Autodesk Fusion 360 part; units mm, degrees
sketch "Sketch1" plane through (0, 0, 0) normal (0, 1, 0) x (1, 0, 0)
  line L0 (0, 0) -> (0, -20)
  line L1 (0, -20) -> (16, -20)
  line L2 (16, -20) -> (16, 0)
  line L3 (16, 0) -> (13, 0)
  line L4 (13, 0) -> (13, -17)
  line L5 (13, -17) -> (3, -17)
  line L6 (3, -17) -> (3, 0)
  line L7 (3, 0) -> (0, 0)
extrude "Extrude1" add sketch "Sketch1" along normal blind 60
sketch "Sketch2" plane through (0, 0, 0) normal (0, -1, 0) x (1, 0, 0)
  line L0 (0, 0) -> (3, 0)
  line L1 (3, 0) -> (3, 17)
  line L2 (3, 17) -> (13, 17)
  line L3 (13, 17) -> (13, 0)
  line L4 (13, 0) -> (16, 0)
  line L5 (16, 0) -> (16, 20)
  line L6 (16, 20) -> (0, 20)
  line L7 (0, 20) -> (0, 0)
  line L8 (16, 0) -> (66, 0)
  line L9 (66, 0) -> (66, 85)
  line L10 (66, 85) -> (146, 85)
  line L11 (146, 85) -> (146, 0)
  line L12 (146, 0) -> (166, 0)
  line L13 (166, 0) -> (166, 205)
  line L14 (166, 205) -> (46, 205)
  line L15 (46, 205) -> (46, 20)
  line L16 (46, 20) -> (16, 20)
  dimension "d3" = 50
  dimension "d4" = 85
  dimension "d5" = 80
  dimension "d6" = 20
  dimension "d7" = 205
  dimension "d8" = 120
  dimension "d9" = 185
extrude "Extrude2" add sketch "Sketch2" against normal blind 3 contours L5 L8 L9 L10 L11 L12 L13 L14 L15 L16
sketch "Sketch3" plane through (0, 0, 0) normal (0, 1, 0) x (1, 0, 0)
  line L0 (65, 0) -> (150, 0)
  line L1 (150, 0) -> (150, -10)
  line L2 (150, -10) -> (65, -10)
  line L3 (65, -10) -> (65, 0)
extrude "Extrude3" add sketch "Sketch3" along normal blind 3
sketch "Sketch4" plane through (0, 0, 0) normal (0, 1, 0) x (1, 0, 0)
sketch "Sketch5" plane through (0, 0, 0) normal (0, 0, 1) x (1, 0, 0)
  line L0 (16, 3) -> (16, 30)
  line L1 (16, 30) -> (43, 3)
  line L2 (43, 3) -> (16, 3)
extrude "Extrude4" add sketch "Sketch5" along normal blind 3
sketch "Sketch6" plane through (0, 0, 0) normal (0, -1, 0) x (1, 0, 0)
  line L0 (66, 10) -> (66, 85)
  line L1 (66, 85) -> (146, 85)
  line L2 (146, 85) -> (146, 10)
  line L3 (146, 10) -> (66, 10)
  line L4 (13, 0) -> (166, 0)
  line L5 (166, 0) -> (166, 205)
  line L6 (166, 205) -> (46, 205)
  line L7 (46, 205) -> (46, 20)
  line L8 (46, 20) -> (16, 20)
  line L9 (16, 20) -> (0, 20)
  line L10 (0, 20) -> (0, 0)
  line L11 (0, 0) -> (3, 0)
  line L12 (3, 0) -> (3, 17)
  line L13 (3, 17) -> (13, 17)
  line L14 (13, 17) -> (13, 0)
  circle A0 centre (51.25, 199.75) radius 2.25
  circle A1 centre (160.75, 199.75) radius 2.25
  circle A2 centre (51.25, 90.25) radius 2.25
  circle A3 centre (160.75, 90.25) radius 2.25
  dimension "d16" = 4.5
  dimension "d17" = 5.25
  dimension "d18" = 5.25
  dimension "d19" = 4.5
  dimension "d20" = 5.25
  dimension "d21" = 5.25
  dimension "d22" = 4.5
  dimension "d23" = 5.25
  dimension "d24" = 114.75
  dimension "d25" = 4.5
  dimension "d26" = 5.25
  dimension "d27" = 114.75
extrude "Extrude5" cut sketch "Sketch6" against normal blind 5 contours A0 | A1 | A2 | A3
sketch "Sketch7" plane through (0, 0, 0) normal (0, -1, 0) x (1, 0, 0)
  circle A0 centre (160.75, 90.25) radius 2.25
  circle A1 centre (160.75, 199.75) radius 2.25
  circle A2 centre (51.25, 90.25) radius 2.25
  circle A3 centre (51.25, 199.75) radius 2.25
  line L0 (66, 10) -> (66, 85)
  line L1 (66, 85) -> (146, 85)
  line L2 (146, 85) -> (146, 10)
  line L3 (146, 10) -> (66, 10)
  line L4 (13, 0) -> (166, 0)
  line L5 (166, 0) -> (166, 205)
  line L6 (166, 205) -> (46, 205)
  line L7 (46, 205) -> (46, 20)
  line L8 (46, 20) -> (16, 20)
  line L9 (16, 20) -> (0, 20)
  line L10 (0, 20) -> (0, 0)
  line L11 (0, 0) -> (3, 0)
  line L12 (3, 0) -> (3, 17)
  line L13 (3, 17) -> (13, 17)
  line L14 (13, 17) -> (13, 0)
  line L15 (51, 185) -> (67, 201)
  line L16 (67, 201) -> (145, 201)
  line L17 (145, 201) -> (160.9711, 185.0289)
  line L18 (160.9711, 185.0289) -> (160.9711, 107.0289)
  line L19 (51, 185) -> (51, 107)
  line L20 (51, 107) -> (66.9997, 91.0003)
  line L21 (66.9997, 91.0003) -> (144.9997, 91.0003)
  line L22 (144.9997, 91.0003) -> (160.9711, 107.0289)
  dimension "d30" = 78
  dimension "d31" = 22.627
  dimension "d32" = 78
  dimension "d33" = 78
extrude "Extrude6" cut sketch "Sketch7" against normal blind 10 contours L15 L16 L17 L18 L19 L20 L21 L22
sketch "Sketch8" plane through (0, 0, 0) normal (0, -1, 0) x (1, 0, 0)
  line L0 (66.9997, 91.0003) -> (51, 107)
  line L1 (51, 107) -> (51, 185)
  line L2 (51, 185) -> (67, 201)
  line L3 (67, 201) -> (145, 201)
  line L4 (145, 201) -> (160.9711, 185.0289)
  line L5 (160.9711, 185.0289) -> (160.9711, 107.0289)
  line L6 (160.9711, 107.0289) -> (144.9997, 91.0003)
  line L7 (144.9997, 91.0003) -> (66.9997, 91.0003)
  circle A0 centre (160.75, 90.25) radius 2.25
  circle A1 centre (160.75, 199.75) radius 2.25
  circle A2 centre (51.25, 90.25) radius 2.25
  line L8 (66, 10) -> (66, 85)
  line L9 (66, 85) -> (146, 85)
  line L10 (146, 85) -> (146, 10)
  line L11 (146, 10) -> (66, 10)
  line L12 (13, 0) -> (166, 0)
  line L13 (166, 0) -> (166, 205)
  line L14 (166, 205) -> (46, 205)
  line L15 (46, 205) -> (46, 20)
  line L16 (46, 20) -> (16, 20)
  line L17 (16, 20) -> (0, 20)
  line L18 (0, 20) -> (0, 0)
  line L19 (0, 0) -> (3, 0)
  line L20 (3, 0) -> (3, 17)
  line L21 (3, 17) -> (13, 17)
  line L22 (13, 17) -> (13, 0)
sketch "Sketch9" plane through (0, 0, 0) normal (0, -1, 0) x (1, 0, 0)
  circle A0 centre (51, 200) radius 3.6056
extrude "Extrude7" add sketch "Sketch9" against normal blind 3
sketch "Sketch10" plane through (0, 0, 0) normal (0, -1, 0) x (1, 0, 0)
  circle A0 centre (53.5, 197.5) radius 2.25
  line L0 (46, 205) -> (46, 20)
  line L1 (166, 205) -> (46, 205)
  dimension "d38" = 4.5
  dimension "d39" = 7.5
  dimension "d40" = 7.5
sketch "Sketch11" plane through (0, 0, 0) normal (0, -1, 0) x (1, 0, 0)
  circle A0 centre (160, 200) radius 4.464
extrude "Extrude8" add sketch "Sketch11" against normal blind 3
sketch "Sketch12" plane through (0, 0, 0) normal (0, -1, 0) x (1, 0, 0)
  circle A0 centre (158.5, 197.5) radius 2.25
  line L0 (166, 0) -> (166, 205)
  line L1 (166, 205) -> (46, 205)
  dimension "d43" = 4.5
  dimension "d44" = 7.5
  dimension "d45" = 7.5
extrude "Extrude9" cut sketch "Sketch10" against normal blind 3
extrude "Extrude10" cut sketch "Sketch12" against normal blind 3
sketch "Sketch13" plane through (0, 0, 0) normal (0, -1, 0) x (1, 0, 0)
  circle A0 centre (50, 90) radius 3.5652
  circle A1 centre (160, 90) radius 4.4009
extrude "Extrude11" add sketch "Sketch13" against normal blind 3 contours A0
extrude "Extrude12" add sketch "Sketch8" against normal blind 3 contours A0
sketch "Sketch14" plane through (0, 0, 0) normal (0, -1, 0) x (1, 0, 0)
  circle A0 centre (158.5, 197.5) radius 2.25
  circle A1 centre (53.5, 197.5) radius 2.25
  line L0 (66.9997, 91.0003) -> (51, 107)
  line L1 (51, 107) -> (51, 185)
  line L2 (51, 185) -> (67, 201)
  line L3 (67, 201) -> (145, 201)
  line L4 (145, 201) -> (160.9711, 185.0289)
  line L5 (160.9711, 185.0289) -> (160.9711, 107.0289)
  line L6 (160.9711, 107.0289) -> (144.9997, 91.0003)
  line L7 (144.9997, 91.0003) -> (66.9997, 91.0003)
  line L8 (66, 10) -> (66, 85)
  line L9 (66, 85) -> (146, 85)
  line L10 (146, 85) -> (146, 10)
  line L11 (146, 10) -> (66, 10)
  line L12 (13, 0) -> (166, 0)
  line L13 (166, 0) -> (166, 205)
  line L14 (166, 205) -> (46, 205)
  line L15 (46, 205) -> (46, 20)
  line L16 (46, 20) -> (16, 20)
  line L17 (16, 20) -> (0, 20)
  line L18 (0, 20) -> (0, 0)
  line L19 (0, 0) -> (3, 0)
  line L20 (3, 0) -> (3, 17)
  line L21 (3, 17) -> (13, 17)
  line L22 (13, 17) -> (13, 0)
  circle A2 centre (53.5, 92.5) radius 2.25
  circle A3 centre (158.5, 92.5) radius 2.25
  dimension "d54" = 4.5
  dimension "d55" = 7.5
  dimension "d57" = 7.5
  dimension "d58" = 4.5
  dimension "d59" = 7.5
  dimension "d60" = 7.5
extrude "Extrude13" cut sketch "Sketch14" against normal blind 3 contours A2 | A3
fillet "Fillet1" radius 5 1 edges at (46, 1.5, 205)
fillet "Fillet2" radius 5 1 edges at (166, 1.5, 205)
fillet "Fillet3" radius 5 1 edges at (166, 1.5, 0)
extrude "Extrude14" add 1 faces at (59.3333, 3, 38.3333) along direction (0, 1, 0) blind 2
sketch "Sketch15" plane through (0, 5, 0) normal (0, 1, 0) x (-1, 0, 0)
  arc A0 (-166, 5) -> (-161, 0) centre (-161, 5) ccw
  line L0 (-161, 0) -> (-43, 0)
  line L1 (-43, 0) -> (-43, 3)
  line L2 (-43, 3) -> (-41, 3)
  line L3 (-41, 3) -> (-16, 3)
  line L4 (-16, 3) -> (-16, 20)
  line L5 (-16, 20) -> (-46, 20)
  line L6 (-46, 20) -> (-46, 200)
  arc A1 (-46, 200) -> (-51, 205) centre (-51, 200) ccw
  line L7 (-51, 205) -> (-161, 205)
  arc A2 (-161, 205) -> (-166, 200) centre (-161, 200) ccw
  line L8 (-166, 200) -> (-166, 5)
  circle A3 centre (-53.5, 92.5) radius 2.25
  circle A4 centre (-158.5, 92.5) radius 2.25
  circle A5 centre (-158.5, 197.5) radius 2.25
  circle A6 centre (-53.5, 197.5) radius 2.25
  line L9 (-51, 107) -> (-66.9997, 91.0003)
  line L10 (-66.9997, 91.0003) -> (-144.9997, 91.0003)
  line L11 (-144.9997, 91.0003) -> (-160.9711, 107.0289)
  line L12 (-160.9711, 107.0289) -> (-160.9711, 185.0289)
  line L13 (-160.9711, 185.0289) -> (-145, 201)
  line L14 (-145, 201) -> (-67, 201)
  line L15 (-67, 201) -> (-51, 185)
  line L16 (-51, 185) -> (-51, 107)
  line L17 (-66, 10) -> (-146, 10)
  line L18 (-146, 10) -> (-146, 85)
  line L19 (-146, 85) -> (-66, 85)
  line L20 (-66, 85) -> (-66, 10)
  line L21 (-166, 10.0934) -> (-16, 10.0934)
  line L22 (-16, 10.0934) -> (-16, 5.0934)
  line L23 (-16, 5.0934) -> (-166, 5.0934)
  line L24 (-166, 5.0934) -> (-166, 10.0934)
  dimension "d71" = 5
extrude "Extrude15" add sketch "Sketch15" along normal blind 10 contours L4 L8 L17 L18 L20 L21 L22 L23 L24
sketch "Sketch16" plane through (0, 5, 0) normal (0, 1, 0) x (-1, 0, 0)
  line L0 (-166, 10.0934) -> (-146, 10.0934)
  line L1 (-146, 10.0934) -> (-146, 85)
  line L2 (-146, 85) -> (-66, 85)
  line L3 (-66, 85) -> (-66, 10.0934)
  line L4 (-66, 10.0934) -> (-16, 10.0934)
  line L5 (-16, 10.0934) -> (-16, 20)
  line L6 (-16, 20) -> (-46, 20)
  line L7 (-46, 20) -> (-46, 200)
  arc A0 (-46, 200) -> (-51, 205) centre (-51, 200) ccw
  line L8 (-51, 205) -> (-161, 205)
  arc A1 (-161, 205) -> (-166, 200) centre (-161, 200) ccw
  line L9 (-166, 200) -> (-166, 10.0934)
  line L10 (-51, 107) -> (-66.9997, 91.0003)
  line L11 (-66.9997, 91.0003) -> (-144.9997, 91.0003)
  line L12 (-144.9997, 91.0003) -> (-160.9711, 107.0289)
  line L13 (-160.9711, 107.0289) -> (-160.9711, 185.0289)
  line L14 (-160.9711, 185.0289) -> (-145, 201)
  line L15 (-145, 201) -> (-67, 201)
  line L16 (-67, 201) -> (-51, 185)
  line L17 (-51, 185) -> (-51, 107)
  circle A2 centre (-53.5, 197.5) radius 2.25
  circle A3 centre (-158.5, 197.5) radius 2.25
  circle A4 centre (-158.5, 92.5) radius 2.25
  circle A5 centre (-53.5, 92.5) radius 2.25
  line L18 (-158.5, 10.0934) -> (-153.5, 10.0934)
  line L19 (-153.5, 10.0934) -> (-153.5, 85.0934)
  line L20 (-153.5, 85.0934) -> (-158.5, 85.0934)
  line L21 (-158.5, 85.0934) -> (-158.5, 10.0934)
  dimension "d74" = 75
  dimension "d75" = 7.5
  dimension "d76" = 5
extrude "Extrude16" add sketch "Sketch16" along normal blind 10 contours L0 L18 L19 L20 L21
sketch "Sketch17" plane through (0, 5, 0) normal (0, 1, 0) x (-1, 0, 0)
  circle A0 centre (-53.5, 92.5) radius 2.25
  circle A1 centre (-158.5, 92.5) radius 2.25
  circle A2 centre (-158.5, 197.5) radius 2.25
  circle A3 centre (-53.5, 197.5) radius 2.25
  line L0 (-51, 107) -> (-66.9997, 91.0003)
  line L1 (-66.9997, 91.0003) -> (-144.9997, 91.0003)
  line L2 (-144.9997, 91.0003) -> (-160.9711, 107.0289)
  line L3 (-160.9711, 107.0289) -> (-160.9711, 185.0289)
  line L4 (-160.9711, 185.0289) -> (-145, 201)
  line L5 (-145, 201) -> (-67, 201)
  line L6 (-67, 201) -> (-51, 185)
  line L7 (-51, 185) -> (-51, 107)
  line L8 (-158.5, 10.0934) -> (-158.5, 85.0934)
  line L9 (-158.5, 85.0934) -> (-153.5, 85.0934)
  line L10 (-153.5, 85.0934) -> (-153.5, 10.0934)
  line L11 (-153.5, 10.0934) -> (-146, 10.0934)
  line L12 (-146, 10.0934) -> (-146, 85)
  line L13 (-146, 85) -> (-66, 85)
  line L14 (-66, 85) -> (-66, 10.0934)
  line L15 (-66, 10.0934) -> (-16, 10.0934)
  line L16 (-16, 10.0934) -> (-16, 20)
  line L17 (-16, 20) -> (-46, 20)
  line L18 (-46, 20) -> (-46, 200)
  arc A4 (-46, 200) -> (-51, 205) centre (-51, 200) ccw
  line L19 (-51, 205) -> (-161, 205)
  arc A5 (-161, 205) -> (-166, 200) centre (-161, 200) ccw
  line L20 (-166, 200) -> (-166, 10.0934)
  line L21 (-166, 10.0934) -> (-158.5, 10.0934)
  line L22 (-58.5, 10.0934) -> (-53.5, 10.0934)
  line L23 (-53.5, 10.0934) -> (-53.5, 85.0934)
  line L24 (-53.5, 85.0934) -> (-58.5, 85.0934)
  line L25 (-58.5, 85.0934) -> (-58.5, 10.0934)
  dimension "d79" = 5
  dimension "d80" = 75
  dimension "d81" = 7.5
extrude "Extrude17" add sketch "Sketch17" along normal blind 10 contours L15 L22 L23 L24 L25
extrude "Extrude18" add 1 faces at (1, 60, 12.3333) along direction (0, 1, 0) blind 30
Design review of the part built by this model. Coordinates are the model's own, in mm. A direction names the side the tool comes from. Round coordinates to 2 decimals unless told otherwise and drop trailing zeros. Loops run counter-clockwise (first coordinate to the right, second up) from the corner with the lowest first, then second, coordinate; pieces in that order, holes last. Notation, with made-up numbers: (15, 54) -> (74, 54) arc R7 cw to (74, 67) -> close; hole circle Ø7 at (-30.75, -15). An arc over 180 degrees is marked (long way). Use one line per item in the form item = value. Start each with the question number.
Q1. Wall thickness on line 1 along Z through (x, y) = (158.5, 2.5); line 2 along Z through (x, y) = (158, 3); line 3 along Y through (x, z) = (68.5, 88): over which ranges is each line inside the solid? List them lowest first. Write a range as [from, to].
Q2. For pin 1 Ø1.6 at (x, y) = (42, 3.5) entering from -Z; pin 2 Ø5 at (y, z) = (8, 38.5) entering from -X; pin 3 Ø4.5 at (y, z) = (4.5, 65) entering from -X; pin 4 Ø2 at (x, y) = (150, 9.5) entering from +Z, all flat-tipped, find the tip position at first contact; note any pin that passes through.
Q3. We need section D-D on y = 67. Give the boundary of the cut face in (x, z), then the cut area to 3 significant figures.
Q4. We need section C-C on z = 48.5. Give the boundary of the cut face in (x, y), then the cut area to 3 significant figures.
Q5. Draft analysis for pull direction Z (two halves, no side actions). For faces 1 (the face through (13, 44, 8)), 2 (the face through (56, 10, 85.093)), 3 (the face through (51.714, 2.465, 91.131)), state which applies: +Z half, -Z half, draft (parallel to the pull), parting line (faces both ways), or undercut.
Q6. We need section A-A on z = 197.5. Give the boundary of the cut face in (x, y), then the cut area to 3 significant figures.
Q7. We need section B-B on x = 131.5. Give the boundary of the cut face in (y, z), then the cut area to 3 significant figures.
Q8. Machinability: for faces 4 (the face through (35, 10, 10.093)), 5 (the face through (8, 44, 17)), 6 (the face through (146, 2, 47)), which of the approach directions +Z, -Z, +X, -X, +Y, -Y give a long, thin tool a straight path to every point of the face, cutting with its end or side? Answer none if there is none.
Calculated:
q1.line_1 = [0, 90.25], [94.75, 104.55], [187.5, 195.25], [199.75, 205]
q1.line_2 = [0, 90.31], [94.69, 104.05], [188, 195.31], [199.69, 205]
q1.line_3 = [0, 5]
q2.pin_1 = 0
q2.pin_2 = 53.5
q2.pin_3 = 46
q2.pin_4 = 10.09
q3.outline = (0, 0) -> (3, 0) -> (3, 17) -> (13, 17) -> (13, 0) -> (16, 0) -> (16, 20) -> (0, 20) -> close
q3.area = 150 mm²
q4.outline = (46, 0) -> (66, 0) -> (66, 5) -> (58.5, 5) -> (58.5, 15) -> (53.5, 15) -> (53.5, 5) -> (46, 5) -> close; (146, 0) -> (166, 0) -> (166, 5) -> (158.5, 5) -> (158.5, 15) -> (153.5, 15) -> (153.5, 5) -> (146, 5) -> close
q4.area = 300 mm²
q5.face_1 = draft
q5.face_2 = +Z half
q5.face_3 = undercut
q6.outline = (46, 0) -> (51.25, 0) -> (51.25, 5) -> (46, 5) -> close; (55.75, 0) -> (63.5, 0) -> (63.5, 5) -> (55.75, 5) -> close; (148.5, 0) -> (156.25, 0) -> (156.25, 5) -> (148.5, 5) -> close; (160.75, 0) -> (166, 0) -> (166, 5) -> (160.75, 5) -> close
q6.area = 130 mm²
q7.outline = (0, 0) -> (5, 0) -> (5, 5.09) -> (15, 5.09) -> (15, 10) -> (0, 10) -> close; (0, 85) -> (5, 85) -> (5, 91) -> (0, 91) -> close; (0, 201) -> (5, 201) -> (5, 205) -> (0, 205) -> close
q7.area = 149 mm²
q8.face_4 = +Z, +Y
q8.face_5 = -Z, +Y, -Y
q8.face_6 = +Y, -Y
